Part model, mm, in its own coordinate system. Face numbers are marked on the shaded views. A direction names the side the tool comes from. Give positions to 0.01 mm unless a question says otherwise; leave off trailing zeros. Order: outer loops, then holes, each group sorted by start corner. A loop starts at its lowest first (then second) coordinate and runs counter-clockwise, first axis right, second up. Notation, with made-up numbers: M 87.25,39.25 L 113.25,39.25 A14 ccw 113.25,58.25 Z; hole C 17,-39.5 d9. An arc over 180 degrees is marked long. Answer as a JSON object with one key per item and string values.
from build123d import *

# Parameters (mm, degrees)
BOSS_EXTRU_1_DEPTH      = 3
ESQUISSE2_R             = 1.25
ENL_V_MAT_EXTRU_1_DEPTH = 7
CONG_2_R                = 0.5


with BuildPart() as part:
    # Esquisse1 → Boss.-Extru.1 (new body, symmetric)
    with BuildSketch(Plane.XY):
        Polygon((-6, 0), (-2.4, 0), (-2.4, -3.5), (2.4, -3.5), (2.4, 0), (6, 0), (6, 2.5), (-6, 2.5), align=None)
    extrude(amount=BOSS_EXTRU_1_DEPTH, both=True)

    # Esquisse2 → Enlèv. mat.-Extru.1 (cut, through all)
    with BuildSketch(Plane(origin=(0, 2.5, 0), x_dir=(1, 0, 0), z_dir=(0, 1, 0))):
        Circle(ESQUISSE2_R)
    extrude(amount=-ENL_V_MAT_EXTRU_1_DEPTH, mode=Mode.SUBTRACT)

    # Congé2
    cong_2_edges = [part.edges().sort_by_distance(p)[0] for p in [
        (-6, 1.25, -3),
        (6, 1.25, -3),
        (-6, 1.25, 3),
        (-2.4, -1.75, 3),
        (2.4, -1.75, 3),
        (6, 1.25, 3),
        (2.4, -1.75, -3),
        (-2.4, -1.75, -3),
    ]]
    fillet(cong_2_edges, radius=CONG_2_R)


solid = part.part
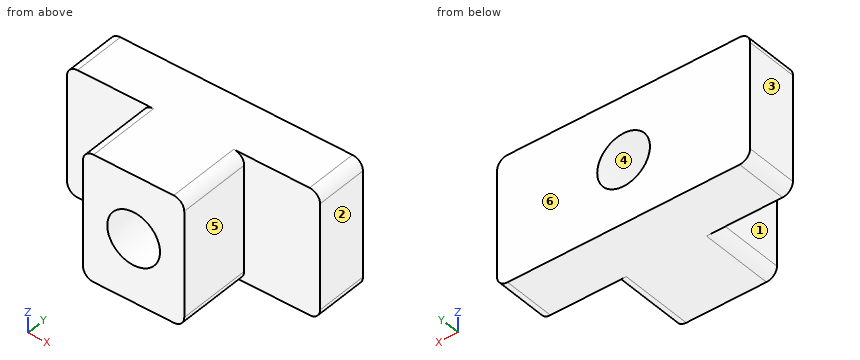
1. Cut at B-B on z = 0. Give the cut face in (x, y).
Worked answers:
{"outline": "M -6,0 L -2.4,0 L -2.4,-3.5 L -1.25,-3.5 L -1.25,2.5 L -6,2.5 Z; M 1.25,-3.5 L 2.4,-3.5 L 2.4,0 L 6,0 L 6,2.5 L 1.25,2.5 Z"}
2. Two-plate mould, pull along X, no slides. Class the marked faces 3, 4, 5 and 6: +X half, -X half, draft (parallel to the pull), parting line (faces both ways), or undercut.
Worked answers:
{"face 3": "-X half", "face 4": "undercut", "face 5": "+X half", "face 6": "draft"}
3. Cut at A-A on x = 0. Give the cut face in (y, z).
Worked answers:
{"outline": "M -3.5,-3 L 2.5,-3 L 2.5,-1.25 L -3.5,-1.25 Z; M -3.5,1.25 L 2.5,1.25 L 2.5,3 L -3.5,3 Z"}
4. Probe line 1 along X through (y, z) = (0.05, 0); line 2 along X through (y, z) = (-1, 0); line 3 along Z through (x, y) = (0, 0.3). List the from-to ranges inside material, lowest first.
Worked answers:
{"line 1": "x = -6 to -1.25, 1.25 to 6", "line 2": "x = -2.4 to -1.25, 1.25 to 2.4", "line 3": "z = -3 to -1.25, 1.25 to 3"}
5. Pin check, flat tips, straight feed: P1, Ø3, axis at y = -2.5, z = -0.5, coming from the +X side; P2, Ø1.8, axis at y = -1.5, z = 0, coming from the -X side. Stop position of each tip, or through.
Worked answers:
{"P1": "stops at x = 2.4", "P2": "stops at x = -2.4"}
6. Cut at C-C on y = 0.65. Give the cut face in (x, z).
Worked answers:
{"outline": "M -6,-2.5 A0.5 ccw -5.5,-3 L 5.5,-3 A0.5 ccw 6,-2.5 L 6,2.5 A0.5 ccw 5.5,3 L -5.5,3 A0.5 ccw -6,2.5 Z; hole C 0,0 d2.5"}
7. Cut at D-D on y = -1.4. Give the cut face in (x, z), plus the area to 3 significant figures.
Worked answers:
{"outline": "M -2.4,-2.5 A0.5 ccw -1.9,-3 L 1.9,-3 A0.5 ccw 2.4,-2.5 L 2.4,2.5 A0.5 ccw 1.9,3 L -1.9,3 A0.5 ccw -2.4,2.5 Z; hole C 0,0 d2.5", "area": "23.7 mm^2"}
8. Which spindle directions (+Z, -Z, +X, -X, +Y, -Y) get a long thin tool onto all of the face, cutting with end or side? Do the marked faces 1 and 2. Say none if no direction does.
Worked answers:
{"face 1": "+Z, -Z, -X, -Y", "face 2": "+Z, -Z, +X, +Y, -Y"}
